Can you work these out from the drawing? Everything is in mm from the part's minimum corner. Round coordinates to 2 decimals unless told otherwise and drop trailing zeros. Loops run counter-clockwise (first coordinate to the right, second up) from the corner with the lowest first, then second, coordinate; pieces in that order, holes last. Notation, with made-up numbers: (-32, -22) -> (-11, -22) arc R16 ccw to (-11, -9) -> close; hole circle Ø7 at (44.5, -38). An arc over 180 degrees is marked (long way). One line per item, written item: value.
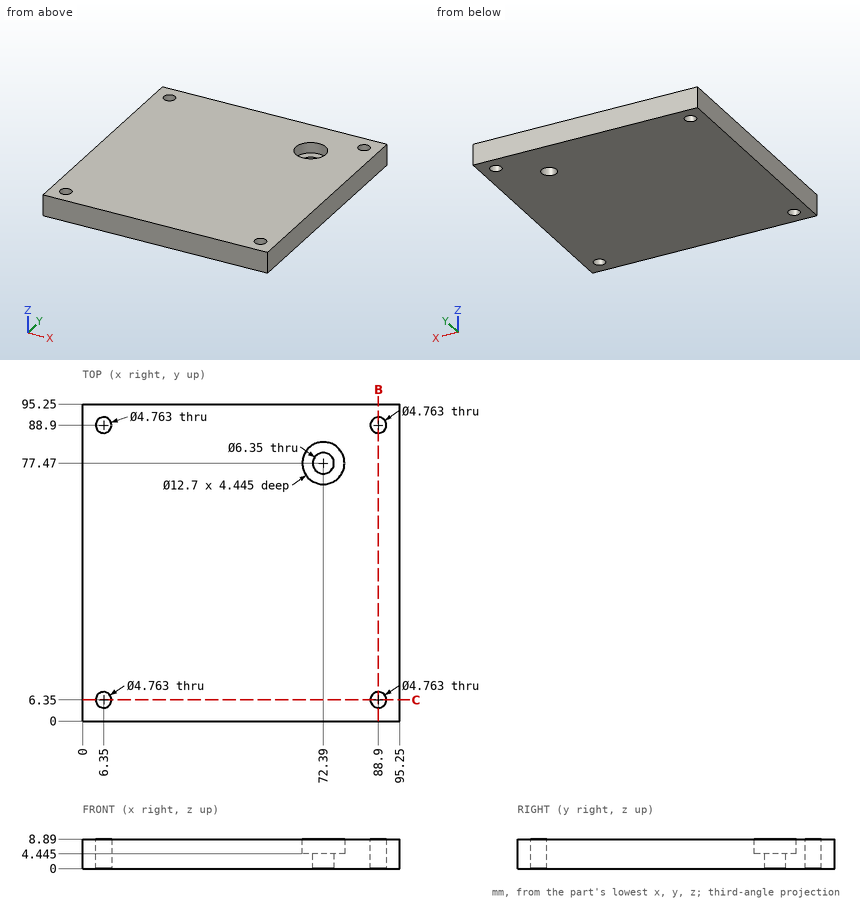
(1) If I drill on L1, parallel to X at y = 88.9, z = 5.5, over which ranges is the centre line in solid material (lowest first)?
Recorded:
L1: 0 to 3.97, 8.73 to 86.52, 91.28 to 95.25
(2) I'm going to push a flat-ended pin straight in: pin 1 Ø11.5 at (x, y) = (72.39, 77.47) entering from +Z (1 decimal). Where does the tip first touch, or does it pass through?
Recorded:
pin 1: z = 4.4
(3) If we section it at B-B, the plane x = 88.9: Please give me the cut outline in (y, z), then the cut area to 3 significant figures.
Recorded:
outline: (0, 0) -> (3.97, 0) -> (3.97, 8.89) -> (0, 8.89) -> close; (8.73, 0) -> (86.52, 0) -> (86.52, 8.89) -> (8.73, 8.89) -> close; (91.28, 0) -> (95.25, 0) -> (95.25, 8.89) -> (91.28, 8.89) -> close
area: 762 mm²
